from build123d import *

# Parameters (mm, degrees)
SKETCH_2_W          = 45.085
SKETCH_2_H          = 100.076
EXTRUDE_1_DEPTH     = 1.6
SKETCH_3_W          = 3.6000436
SKETCH_3_H          = 6.0999624
EXTRUDE_2_DEPTH     = 2.5
SKETCH_4_W          = 35.0519492
SKETCH_4_H          = 7.9370174
EXTRUDE_3_DEPTH     = 6.5
SKETCH_5_W          = 8
SKETCH_5_H          = 4.5
EXTRUDE_4_DEPTH     = 14
SKETCH_6_W          = 11.999976
SKETCH_6_H          = 11.999976
EXTRUDE_5_DEPTH     = 12.7
SKETCH_8_W          = 11.69819953
SKETCH_8_H          = 11.69819953
EXTRUDE_8_DEPTH     = 2
SKETCH_9_R          = 1.599946
CUT_EXTRUDE_1_DEPTH = 2
SKETCH_10_R         = 3.81
EXTRUDE_9_DEPTH     = 8
SKETCH_11_W         = 5.969
SKETCH_11_H         = 31.369
EXTRUDE_10_DEPTH    = 4
SKETCH_12_W         = 3.81
SKETCH_12_H         = 4.800092
EXTRUDE_11_DEPTH    = 2
SKETCH_13_R         = 3.1496
EXTRUDE_12_DEPTH    = 7
SKETCH_14_W         = 2.7701748
SKETCH_14_H         = 1.3212064
EXTRUDE_13_DEPTH    = 1
SKETCH_15_W         = 5.0524156
SKETCH_15_H         = 5.0524156
EXTRUDE_14_DEPTH    = 4


with BuildPart() as part:
    # 草图2 → 凸台-拉伸1 (new body)
    with BuildSketch(Plane.XY):
        with Locations((22.5425, 50.038)):
            Rectangle(SKETCH_2_W, SKETCH_2_H)
    extrude(amount=EXTRUDE_1_DEPTH)

    # 草图3 → 凸台-拉伸2 (add)
    with BuildSketch(Plane.XY.offset(1.6)):
        with Locations((3.81, 95.631)):
            Rectangle(SKETCH_3_W, SKETCH_3_H)
        with Locations((9.906, 95.631)):
            Rectangle(SKETCH_3_W, SKETCH_3_H)
        with Locations((3.81, 86.995)):
            Rectangle(SKETCH_3_W, SKETCH_3_H)
        with Locations((9.906, 86.995)):
            Rectangle(SKETCH_3_W, SKETCH_3_H)
    extrude(amount=EXTRUDE_2_DEPTH)

    # 草图4 → 凸台-拉伸3 (add)
    with BuildSketch(Plane.XY.offset(1.6)):
        with Locations((18.923, 78.5815421)):
            Rectangle(SKETCH_4_W, SKETCH_4_H)
        with Locations((18.923, 69.8185421)):
            Rectangle(SKETCH_4_W, SKETCH_4_H)
        with Locations((18.923, 60.9285421)):
            Rectangle(SKETCH_4_W, SKETCH_4_H)
        with Locations((18.923, 52.0385421)):
            Rectangle(SKETCH_4_W, SKETCH_4_H)
    extrude(amount=EXTRUDE_3_DEPTH)

    # 草图5 → 凸台-拉伸4 (add)
    with BuildSketch(Plane.XY.offset(8.1)):
        with Locations((10.046059562, 78.5815421)):
            Rectangle(SKETCH_5_W, SKETCH_5_H)
        with Locations((10.047675227, 69.8185421)):
            Rectangle(SKETCH_5_W, SKETCH_5_H)
        with Locations((10.046401334, 60.9285421)):
            Rectangle(SKETCH_5_W, SKETCH_5_H)
        with Locations((10.054884801, 52.0385421)):
            Rectangle(SKETCH_5_W, SKETCH_5_H)
    extrude(amount=EXTRUDE_4_DEPTH)

    # 草图6 → 凸台-拉伸5 (add)
    with BuildSketch(Plane.XY.offset(1.6)):
        with Locations((20.193, 91.313)):
            Rectangle(SKETCH_6_W, SKETCH_6_H)
    extrude(amount=EXTRUDE_5_DEPTH)

    # 草图8 → 凸台-拉伸8 (add)
    with BuildSketch(Plane.XY.offset(14.3)):
        with Locations((20.198016327, 91.323022246)):
            Rectangle(SKETCH_8_W, SKETCH_8_H)
    extrude(amount=EXTRUDE_8_DEPTH)

    # 草图9 → 切除-拉伸1 (cut)
    with BuildSketch(Plane.XY.offset(1.6)):
        with Locations((38.735, 87.376)):
            Circle(SKETCH_9_R)
        with Locations((29.591, 2.794)):
            Circle(SKETCH_9_R)
        with Locations((11.43, 2.794)):
            Circle(SKETCH_9_R)
    extrude(amount=-CUT_EXTRUDE_1_DEPTH, mode=Mode.SUBTRACT)

    # 草图10 → 凸台-拉伸9 (add)
    with BuildSketch(Plane.XY.offset(1.6)):
        with Locations((5.588, 13.589)):
            Circle(SKETCH_10_R)
        with Locations((14.732, 13.589)):
            Circle(SKETCH_10_R)
        with Locations((23.495, 13.462)):
            Circle(SKETCH_10_R)
        with Locations((32.385, 13.335)):
            Circle(SKETCH_10_R)
    extrude(amount=EXTRUDE_9_DEPTH)

    # 草图11 → 凸台-拉伸10 (add)
    with BuildSketch(Plane.XY.offset(1.6)):
        with Locations((40.8305, 64.8335)):
            Rectangle(SKETCH_11_W, SKETCH_11_H)
    extrude(amount=EXTRUDE_10_DEPTH)

    # 草图12 → 凸台-拉伸11 (add)
    with BuildSketch(Plane.XY.offset(1.6)):
        with Locations((11.303, 41.783)):
            Rectangle(SKETCH_12_W, SKETCH_12_H)
        with Locations((11.303, 34.798)):
            Rectangle(SKETCH_12_W, SKETCH_12_H)
        with Locations((11.303, 27.813)):
            Rectangle(SKETCH_12_W, SKETCH_12_H)
        with Locations((11.303, 20.701)):
            Rectangle(SKETCH_12_W, SKETCH_12_H)
    extrude(amount=EXTRUDE_11_DEPTH)

    # 草图13 → 凸台-拉伸12 (add)
    with BuildSketch(Plane.XY.offset(1.6)):
        with Locations((3.683, 42.418)):
            Circle(SKETCH_13_R)
        with Locations((3.683, 35.433)):
            Circle(SKETCH_13_R)
        with Locations((3.556, 28.448)):
            Circle(SKETCH_13_R)
        with Locations((3.556, 21.336)):
            Circle(SKETCH_13_R)
        with Locations((40.386, 44.45)):
            Circle(SKETCH_13_R)
        with Locations((40.386, 37.719)):
            Circle(SKETCH_13_R)
        with Locations((40.386, 30.48)):
            Circle(SKETCH_13_R)
        with Locations((40.386, 22.86)):
            Circle(SKETCH_13_R)
    extrude(amount=EXTRUDE_12_DEPTH)

    # 草图14 → 凸台-拉伸13 (add)
    with BuildSketch(Plane.XY.offset(1.6)):
        with Locations((18.923, 44.45)):
            Rectangle(SKETCH_14_W, SKETCH_14_H)
        with Locations((18.923, 42.926)):
            Rectangle(SKETCH_14_W, SKETCH_14_H)
        with Locations((18.923, 41.402)):
            Rectangle(SKETCH_14_W, SKETCH_14_H)
        with Locations((18.923, 39.878)):
            Rectangle(SKETCH_14_W, SKETCH_14_H)
        with Locations((18.923, 37.465)):
            Rectangle(SKETCH_14_W, SKETCH_14_H)
        with Locations((18.923, 35.941)):
            Rectangle(SKETCH_14_W, SKETCH_14_H)
        with Locations((18.923, 34.417)):
            Rectangle(SKETCH_14_W, SKETCH_14_H)
        with Locations((18.923, 32.893)):
            Rectangle(SKETCH_14_W, SKETCH_14_H)
        with Locations((18.923, 30.48)):
            Rectangle(SKETCH_14_W, SKETCH_14_H)
        with Locations((18.923, 18.923)):
            Rectangle(SKETCH_14_W, SKETCH_14_H)
        with Locations((18.923, 20.447)):
            Rectangle(SKETCH_14_W, SKETCH_14_H)
        with Locations((18.923, 21.971)):
            Rectangle(SKETCH_14_W, SKETCH_14_H)
        with Locations((18.923, 23.622)):
            Rectangle(SKETCH_14_W, SKETCH_14_H)
        with Locations((18.923, 25.908)):
            Rectangle(SKETCH_14_W, SKETCH_14_H)
        with Locations((18.923, 27.432)):
            Rectangle(SKETCH_14_W, SKETCH_14_H)
        with Locations((18.923, 28.956)):
            Rectangle(SKETCH_14_W, SKETCH_14_H)
    extrude(amount=EXTRUDE_13_DEPTH)

    # 草图15 → 凸台-拉伸14 (add)
    with BuildSketch(Plane.XY.offset(1.6)):
        with Locations((26.416, 42.545)):
            Rectangle(SKETCH_15_W, SKETCH_15_H)
        with Locations((26.416, 35.56)):
            Rectangle(SKETCH_15_W, SKETCH_15_H)
        with Locations((26.416, 28.575)):
            Rectangle(SKETCH_15_W, SKETCH_15_H)
        with Locations((26.416, 21.717)):
            Rectangle(SKETCH_15_W, SKETCH_15_H)
    extrude(amount=EXTRUDE_14_DEPTH)


solid = part.part
Could you check a few things on this model? Use its own coordinates, in mm. A direction names the side the tool comes from. Give positions to 0.01 mm unless a question says otherwise; leave off trailing zeros. Write each loop counter-clockwise with the first axis right and the second up, starting at its lowest first coordinate (ties: lowest second). Pieces come first, ordered by that corner, then holes. Notation, with made-up numbers: (24, -0.75) -> (32, -0.75) arc R18 cw to (32, 15.25) -> close; hole circle Ø11 at (-35, 46). An arc over 180 degrees is marked (long way). Write each question's results on one line, items separated by ' | '. Start each with the question number.
Q1. We'd pull the mould along Y, two halves only. Please class faces 5 (the face through (20, 97.313, 8)), 6 (the face through (1.397, 61, 5)), 7 (the face through (26, 45.071, 4)): +Y half, -Y half, draft (parallel to the pull), parting line (faces both ways), or undercut.
Q2. Which directions (+Z, -Z, +X, -X, +Y, -Y) give clear straight access to the entire face, cutting with the end or side of a thin tool? Please do faces 1 (the face through (14.349, 91, 15)), 2 (the face through (19, 56.007, 5)), 3 (the face through (43.815, 65, 4)), 4 (the face through (13.208, 35, 3)).
Q3. Suppose I cut it at A-A, the plane y = 94. List the corners of the cut face in (x, z) for me (3 decimals), and give its area (3 significant figures).
Q4. I'm going to push flat-ended pins straight in: pin 1 Ø3 at (x, z) = (39.5, 3.5) entering from -Y; pin 2 Ø8 at (x, z) = (29, 19.5) entering from -Y; pin 3 Ø0.5 at (y, z) = (20.5, 2) entering from -X; pin 4 Ø3 at (y, z) = (79.5, 6) entering from -X. Where does each tip first touch, or does it pass through?
Q5. I need wall thicknesses on probe 1 along X at (y, z) = (94.5, 2.25); probe 2 along Y at (x, z) = (7, 15); probe 3 along Y at (x, z) = (38.5, 2). Which ranges of each line are inside material? Lowest first, please.
Outcome:
1) face 5: +Y half | face 6: draft | face 7: undercut
2) face 1: +Z, -X, +Y, -Y | face 2: +Z, -X | face 3: +Z, +X, +Y, -Y | face 4: +Z
3) outline: (0, 0) -> (45.085, 0) -> (45.085, 1.6) -> (26.193, 1.6) -> (26.193, 14.3) -> (26.047, 14.3) -> (26.047, 16.3) -> (14.349, 16.3) -> (14.349, 14.3) -> (14.193, 14.3) -> (14.193, 1.6) -> (11.706, 1.6) -> (11.706, 4.1) -> (8.106, 4.1) -> (8.106, 1.6) -> (5.61, 1.6) -> (5.61, 4.1) -> (2.01, 4.1) -> (2.01, 1.6) -> (0, 1.6) -> close | area: 266 mm2
4) pin 1: y = 19.71 | pin 2: through | pin 3: x = 0.46 | pin 4: x = 1.4
5) probe 1: 2.01 to 5.61, 8.11 to 11.71, 14.19 to 26.19 | probe 2: 49.79 to 54.29, 58.68 to 63.18, 67.57 to 72.07, 76.33 to 80.83 | probe 3: 20.34 to 25.38, 27.96 to 33, 35.2 to 40.24, 41.93 to 46.97, 49.15 to 80.52
